Here's the drawing with two shaded views (mm, measured from the low corner). I have some questions. Round coordinates to 2 decimals unless told otherwise and drop trailing zeros. Loops run counter-clockwise (first coordinate to the right, second up) from the corner with the lowest first, then second, coordinate; pieces in that order, holes last.
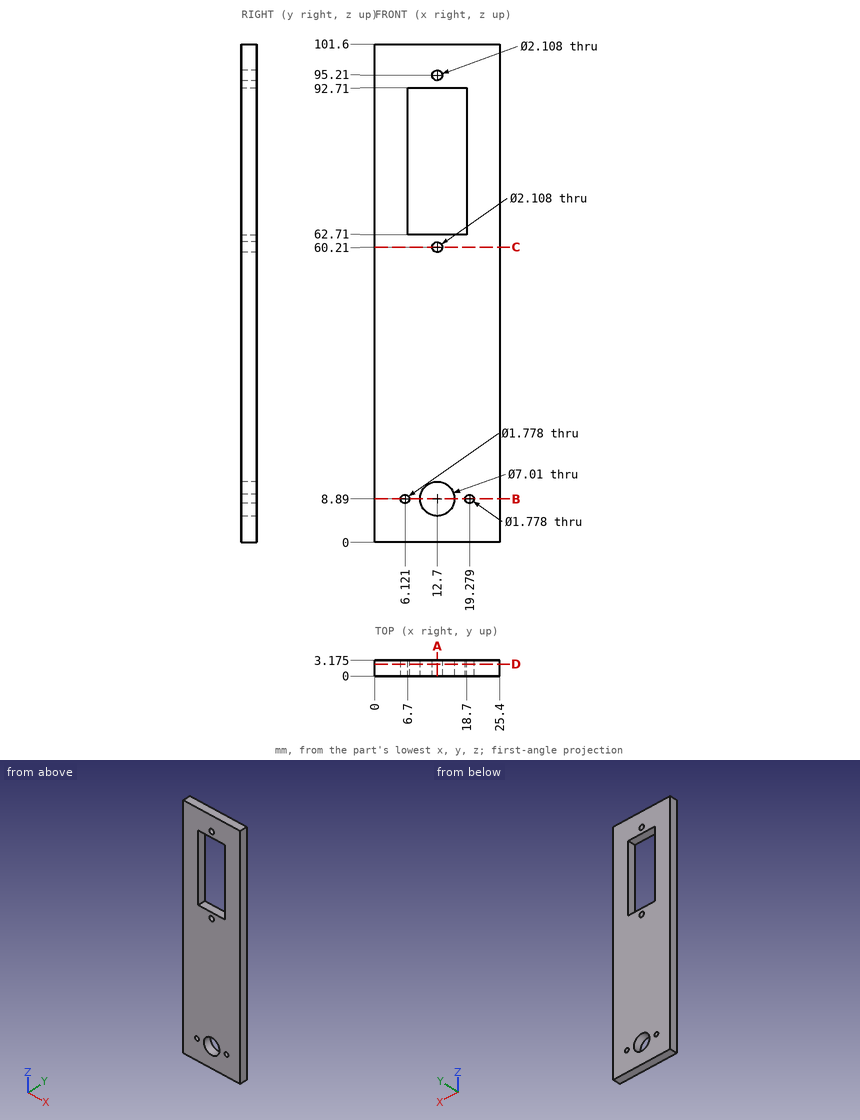
Item 1: If we section it at D-D, the plane y = 2.4: Please give me the cut outline in (x, z) (1 decimal).
Results list:
outline: (0, 0) - (25.4, 0) - (25.4, 101.6) - (0, 101.6) - close; hole circle Ø1.8 at (6.1, 8.9); hole (6.7, 62.7) - (18.7, 62.7) - (18.7, 92.7) - (6.7, 92.7) - close; hole circle Ø7 at (12.7, 8.9); hole circle Ø2.1 at (12.7, 60.2); hole circle Ø2.1 at (12.7, 95.2); hole circle Ø1.8 at (19.3, 8.9)
Item 2: If we section it at A-A, the plane x = 12.7: Please give me the cut outline in (y, z) (1 decimal), then the cut area to 3 significant figures.
Results list:
outline: (0, 0) - (3.2, 0) - (3.2, 5.4) - (0, 5.4) - close; (0, 12.4) - (3.2, 12.4) - (3.2, 59.2) - (0, 59.2) - close; (0, 61.3) - (3.2, 61.3) - (3.2, 62.7) - (0, 62.7) - close; (0, 92.7) - (3.2, 92.7) - (3.2, 94.2) - (0, 94.2) - close; (0, 96.3) - (3.2, 96.3) - (3.2, 101.6) - (0, 101.6) - close
area: 192 mm2
Item 3: Will this pin go through, and if not, where does the flat tip stop? pin 1 (6.5 mm diameter, centred on x = 12.7, z = 8.89, fed in from -Y).
Results list:
pin 1: passes through
Item 4: If we section it at C-C, the plane z = 60.21: Please give me the cut outline in (x, y) (1 decimal).
Results list:
outline: (0, 0) - (11.6, 0) - (11.6, 3.2) - (0, 3.2) - close; (13.8, 0) - (25.4, 0) - (25.4, 3.2) - (13.8, 3.2) - close
Item 5: If we section it at B-B, the plane z = 8.89: Please give me the cut outline in (x, y) (1 decimal).
Results list:
outline: (0, 0) - (5.2, 0) - (5.2, 3.2) - (0, 3.2) - close; (7, 0) - (9.2, 0) - (9.2, 3.2) - (7, 3.2) - close; (16.2, 0) - (18.4, 0) - (18.4, 3.2) - (16.2, 3.2) - close; (20.2, 0) - (25.4, 0) - (25.4, 3.2) - (20.2, 3.2) - close
Item 6: If I drill on line 1 along Z through (x, y) = (12.7, 1.6) (1 decimal); line 2 along X through (y, z) = (1.05, 73.5); line 3 along Z through (x, y) = (17.75, 0.8), over which ranges is the centre line in solid material (lowest first)?
Results list:
line 1: z = 0 to 5.4, 12.4 to 59.2, 61.3 to 62.7, 92.7 to 94.2, 96.3 to 101.6
line 2: x = 0 to 6.7, 18.7 to 25.4
line 3: z = 0 to 62.71, 92.71 to 101.6
